The model under review builds one solid part; all positions refer to its coordinate system, in mm. A direction names the side the tool comes from. Coordinates: 2 decimals unless noted, no trailing zeros. Order: outer loops, then holes, each group sorted by start corner. A loop starts at its lowest first (then second) coordinate and runs counter-clockwise, first axis right, second up. Notation, with made-up numbers: M 15.5,-29 L 73.5,-29 A16 cw 73.5,-24 Z; hole C -10.5,58.25 d7. An arc over 180 degrees is marked long. One line per item, written item: value.
```python
from build123d import *

# Parameters (mm, degrees)
SKETCH2_W = 12.954
SKETCH2_H = 9.525


with BuildPart() as part:
    # Sweep1: sweep along a path in Sketch1
    with BuildLine(Plane(origin=(0, 0, 0), x_dir=(0, 0, -1), z_dir=(1, 0, 0))) as sweep1_path:
        Line((16.54938381, -182.81283345), (82.746919051, -37.764167251))
        ThreePointArc((82.746919051, -37.764167251), (-23.298735464, 87.922430962), (-53.187131299, -73.785594832))
        Line((-53.187131299, -73.785594832), (-16.57165453, -100.179258458))
        ThreePointArc((-16.57165453, -100.179258458), (-10.410929492, -107.954292451), (-9.245359354, -117.80554277))
        Line((-9.245359354, -117.80554277), (-17.963721436, -172.390834655))
        ThreePointArc((-17.963721436, -172.390834655), (-5.258764347, -192.674729259), (16.54938381, -182.81283345))
    # Sketch2 → Sweep1 (sweep)
    with BuildSketch(Plane.XY):
        with Locations((0, 90.957049977)):
            Rectangle(SKETCH2_W, SKETCH2_H)
    sweep(path=sweep1_path.line)


solid = part.part
```
(1) Insertion check: pin 1 Ø4 at (x, z) = (3.5, -20.5) entering from +Y; pin 2 Ø5 at (x, z) = (1.5, 64.5) entering from +Y; pin 3 Ø4 at (x, z) = (-5, 37.5) entering from +Y. Each pin has a flat end and moves straight along its axis. Give the tip position at first contact, or say it passes through.
Geometry results:
pin 1: stops at y = 93.91
pin 2: stops at y = 72.93
pin 3: stops at y = 88.89
(2) We need section B-B, the plane z = 0. State the section outline as (x, y) points.
Geometry results:
outline: M -6.48,-198.21 L 6.48,-198.21 L 6.48,-188.69 L -6.48,-188.69 Z; M -6.48,86.19 L 6.48,86.19 L 6.48,95.72 L -6.48,95.72 Z
(3) Mouldability with a two-part tool opening along Y and no side actions: class faces 4 (the cylindrical face through (-0.091, 93.255, 21.582)), 5 (the flat face through (0.091, -111.25, -54.444)), 6 (the flat face through (-0.091, -107.296, -45.779)) as +Y half, -Y half, draft (parallel to the pull), parting line (faces both ways), or undercut.
Geometry results:
face 4: parting line
face 5: -Y half
face 6: undercut
(4) We need section C-C, the plane x = -3. State the section outline as (y, z) points, plus the area to 3 significant figures.
Geometry results:
outline: M -184.79,-20.88 L -39.74,-87.08 A95.72 ccw long -77.65,55.97 L -104.04,19.36 A13.43 cw -117.05,13.95 L -171.64,22.67 A22.95 ccw Z; hole M -180.84,-12.22 L -35.79,-78.41 A86.19 ccw long -69.92,50.4 L -96.32,13.79 A22.95 cw -118.56,4.54 L -173.14,13.26 A13.43 ccw Z
area: 7,080 mm2
(5) We need section A-A, the plane y = 0. State the section outline as (x, z) points.
Geometry results:
outline: M -6.48,-95.72 L 6.48,-95.72 L 6.48,-86.19 L -6.48,-86.19 Z; M -6.48,86.19 L 6.48,86.19 L 6.48,95.72 L -6.48,95.72 Z
(6) For L1, parallel to Z at x = 0.25, y = 0; L2, parallel to Y at x = 1, z = 0; L3, parallel to Z at x = -3, y = -2.5, list the stretches that pass through material, from the lowest coordinate up.
Geometry results:
L1: z = -95.72 to -86.19, 86.19 to 95.72
L2: y = -198.21 to -188.69, 86.19 to 95.72
L3: z = -95.69 to -86.16, 86.16 to 95.69
(7) Tool access review of faces 1 (the flat face through (0.09, -144.73, 18.37)), 2 (the flat face through (6.477, -67, 55)), 3 (the flat face through (-0.091, -83.304, 31.838)): name each direction out of +Z, -Z, +X, -X, +Y, -Y from which nothing blocks a thin tool from reaching the whole face with its end or side.
Geometry results:
face 1: +Z, +X, -X
face 2: +Z, -Z, +X, +Y, -Y
face 3: +X, -X
